Autodesk Inventor part; units mm, degrees
ref_plane "YZ Plane" through (0, 0, 0) normal (1, 0, 0) x (0, 1, 0)
ref_plane "XZ Plane" through (0, 0, 0) normal (0, 1, 0) x (-1, 0, 0)
ref_plane "XY Plane" through (0, 0, 0) normal (0, 0, 1) x (1, 0, 0)
sketch "スケッチ1" plane through (0, 0, 0) normal (0, 0, 1) x (1, 0, 0)
  line L0 (-59, 0) -> (-38, 0)
  line L1 (-38, 0) -> (-38, -21)
  line L2 (-38, -21) -> (-59, -21)
  line L3 (-59, -21) -> (-59, 0)
  line L4 (-61, 2) -> (-36, 2)
  line L5 (-36, 2) -> (-36, -23)
  line L6 (-36, -23) -> (-61, -23)
  line L7 (-61, -23) -> (-61, 2)
  line L8 (-61, -23) -> (0, -23)
  line L9 (0, -23) -> (0, -17)
  line L10 (0, -17) -> (-61, -17)
  line L11 (-61, -17) -> (-61, -23)
  line L12 (-48.5, -23) -> (-85.5, -23)
  line L13 (-85.5, -23) -> (-85.5, -17)
  line L14 (-85.5, -17) -> (-48.5, -17)
  line L15 (-48.5, -17) -> (-48.5, -23)
  line L16 (-85.5, 1) -> (-82.5, 1)
  line L17 (-82.5, 1) -> (-82.5, -23)
  line L18 (-82.5, -23) -> (-85.5, -23)
  line L19 (-85.5, -23) -> (-85.5, 1)
  line L20 (-85.5, -17) -> (-90.7, -17)
  line L21 (-90.7, -17) -> (-90.7, -23)
  line L22 (-90.7, -23) -> (-85.5, -23)
  line L23 (-85.5, -23) -> (-85.5, -17)
  line L24 (-90.7, -23) -> (-93.7, -23)
  line L25 (-93.7, -23) -> (-93.7, 1)
  line L26 (-93.7, 1) -> (-90.7, 1)
  line L27 (-90.7, 1) -> (-90.7, -23)
  point P0 (0, 0)
  point P1 (-61, -10.5)
  point P2 (-59, -10.5)
  point P3 (-48.5, 2)
  point P4 (-48.5, 0)
  point P5 (-36, -17)
  point P6 (-82.5, -17)
  dimension "d0" = 21
  dimension "d1" = 21
  dimension "d4" = 38
  dimension "d5" = 25
  dimension "d6" = 6
  dimension "d31" = 37
  dimension "d33" = 5.2
  dimension "d34" = 3
  dimension "d35" = 18
extrude "押し出し1" add sketch "スケッチ1" along normal blind 8 contours L10 L9 L8 L5
mirror "ミラー2" about plane through (0, -23, 0) normal (1, 0, 0)
sketch "スケッチ17" plane through (0, 0, 0) normal (0, 0, -1) x (-1, 0, 0)
  line L0 (-15, 13) -> (15, 13)
  line L1 (15, 13) -> (15, -17)
  line L2 (15, -17) -> (-15, -17)
  line L3 (-15, -17) -> (-15, 13)
  line L4 (-36, -17) -> (36, -17)
  point P0 (0, 13)
  point P1 (0, 13)
  point P2 (0, -17)
  dimension "d74" = 30
  dimension "d105" = 30
extrude "押し出し16" add sketch "スケッチ17" against normal blind 18
sketch "スケッチ18" plane through (-15, 13, 0) normal (0, 1, 0) x (1, 0, 0)
  line L0 (5, -15.5) -> (25, -15.5)
  line L1 (25, -15.5) -> (25, -2.5)
  line L2 (25, -2.5) -> (5, -2.5)
  line L3 (5, -2.5) -> (5, -15.5)
  line L4 (0, 0) -> (30, 0)
  line L5 (0, 0) -> (0, -18)
  point P0 (15, 0)
  point P1 (15, -2.5)
  point P2 (15, 0)
  point P3 (5, -9)
  point P4 (0, -9)
  dimension "d77" = 20
  dimension "d78" = 13
extrude "押し出し17" cut sketch "スケッチ18" against normal up to surface (30 mm away)
sketch "スケッチ19" plane through (0, 0, 18) normal (0, 0, 1) x (1, 0, 0)
  line L0 (-15, -17) -> (-15, -23)
  line L1 (15, 13) -> (15, -17)
  line L2 (-15, -17) -> (15, -17)
  line L3 (15, -17) -> (15, 11.5)
  line L4 (15, 11.5) -> (-15, 11.5)
  line L5 (-15, 11.5) -> (-15, -17)
  line L6 (15, 13) -> (-15, 13)
  point P0 (0, 0)
  point P1 (-15, 13)
  point P2 (15, -17)
  dimension "d81" = 1.5
extrude "押し出し18" cut sketch "スケッチ19" against normal up to surface (10 mm away)
sketch "スケッチ20" plane through (-15, 11.5, 8) normal (0, 0, 1) x (1, 0, 0)
  line L0 (0, 0) -> (30, 0)
  line L1 (30, -28.5) -> (51, -28.5)
  line L2 (2.5, 0) -> (47.5, 0)
  line L3 (40.5, -28.5) -> (2.5, -28.5)
  line L4 (2.5, -28.5) -> (2.5, 0)
  line L5 (5, 0) -> (5, -28.5)
  line L6 (25, 0) -> (27.5, 0)
  line L7 (27.5, 0) -> (27.5, -28.5)
  line L8 (27.5, -28.5) -> (25, -28.5)
  line L9 (25, -28.5) -> (25, 0)
  line L10 (25, -28.5) -> (25, 0)
  point P0 (15, -11.5)
  point P1 (40.5, -28.5)
  point P2 (25, -15)
  point P3 (5, -15)
  point P4 (51, -28.5)
  point P5 (5, -16)
  point P6 (25, -28.5)
  point P7 (27.5, 0)
  dimension "d85" = 2.5
  dimension "d113" = 2.5
extrude "押し出し19" cut sketch "スケッチ20" against normal up to surface (5.5 mm away) contours L0 L5 L3 L4 | L0 L7 L3 L9
sketch "スケッチ21" plane through (-10, 13, 2.5) normal (0, 0, 1) x (1, 0, 0)
  line L0 (20, 0) -> (20, -1.5)
  line L1 (0, 0) -> (20, 0)
  line L2 (0, 0) -> (0, -1.5)
  line L3 (-2.5, -30) -> (22.5, -30)
  circle A0 centre (10, -15.75) radius 7.5
  line L4 (-5, -1.5) -> (25, -1.5)
  line L5 (-2.5, -30) -> (-2.5, -1.5)
  line L6 (22.5, -30) -> (22.5, -1.5)
  line L7 (22.5, -1.5) -> (20, -1.5)
  line L8 (0, -1.5) -> (-2.5, -1.5)
  line L9 (-2.5, -1.5) -> (-2.5, -30)
  point P0 (0, -2)
  point P1 (10, -1.5)
  point P2 (25, -1.5)
  point P3 (-2.5, -15.75)
  dimension "d89" = 15
extrude "押し出し20" cut sketch "スケッチ21" against normal through all contours A0
sketch "スケッチ26" plane through (-36, -23, 0) normal (0, -1, 0) x (1, 0, 0)
  line L0 (0, 0) -> (72, 0)
  line L1 (72, 0) -> (72, 8)
  line L2 (0, 8) -> (72, 8)
  line L3 (0, 0) -> (0, 8)
  point P0 (36, 0)
extrude "押し出し25" cut sketch "スケッチ26" against normal up to surface (6 mm away)
sketch "スケッチ27" plane through (-15, -17, 0) normal (0, -1, 0) x (1, 0, 0)
  line L0 (-8.5, 8) -> (38.5, 8)
  line L1 (38.5, 8) -> (38.5, 0)
  line L2 (38.5, 0) -> (-8.5, 0)
  line L3 (-8.5, 0) -> (-8.5, 8)
  line L4 (-5, 8) -> (35, 8)
  line L5 (35, 8) -> (35, 0) construction
  line L6 (35, 0) -> (-5, 0)
  line L7 (-5, 0) -> (-5, 8) construction
  line L8 (0, 8) -> (30, 8)
  line L9 (30, 0) -> (0, 0)
  circle A0 centre (-5, 4) radius 1.6
  circle A1 centre (35, 4) radius 1.6
  point P0 (15, 0)
  point P1 (10.6, 8)
  point P2 (15, 0)
  point P3 (15, 0)
  dimension "d108" = 40
  dimension "d109" = 47
  dimension "d110" = 3.2
extrude "押し出し26" add sketch "スケッチ27" against normal blind 3
fillet "フィレット6" radius 6.5 2 edges at (-15, -14, 4) (15, -14, 4)
sketch "スケッチ28" plane through (-15, -14, 0) normal (0, 1, 0) x (1, 0, 0)
  circle A0 centre (-5, -4) radius 1.6
  circle A1 centre (35, -4) radius 1.6
  line L0 (-8.5, -8) -> (38.5, -8)
  line L1 (-8.5, -8) -> (-8.5, 0)
  line L2 (38.5, 0) -> (-8.5, 0)
  line L3 (38.5, 0) -> (38.5, -8)
  circle A2 centre (35, -4) radius 3
  circle A3 centre (-5, -4) radius 3
  point P0 (15, 0)
  dimension "d116" = 6
extrude "押し出し27" cut sketch "スケッチ28" along normal through all contours A0 | A1 | A2 | A3
fillet "フィレット7" radius 4 4 edges at (-23.5, -15.5, 8) (-23.5, -15.5, 0) (23.5, -15.5, 8) (23.5, -15.5, 0)
fillet "フィレット8" radius 9 2 edges at (12.5, -14, 5.25) (-12.5, -14, 5.25)
equation "\"d0\" = d1"
equation "\"d113\" = d85"
properties part number "スイッチセッター"
Geometry: final body of the model. Coordinates: model frame, mm. A direction names the side the tool comes from. Round coordinates to 2 decimals unless told otherwise and drop trailing zeros. Write each loop counter-clockwise with the first axis right and the second up, starting at its lowest first coordinate (ties: lowest second). Pieces come first, ordered by that corner, then holes. Notation, with made-up numbers: M 16.5,47.5 L 51.5,47.5 A17 cw 51.5,74.5 Z; hole C 79,-38 d1. An arc over 180 degrees is marked long. Answer in a Markdown table with one row per item. Add a question column.
(1) Draft query along Y for faces 1 (the face through (22, -14, 4)), 2 (the face through (0, 12, 15.5)), 3 (the face through (-9.794, -11.434, 5.212)). Return one class per face: pulls with the +Y half, pulls with the -Y half, needs draft (parallel to the pull), parting line crosses it, or undercut.
(2) Reachability of faces 4 (the face through (-21.27, -15.52, 3.03)), 5 (the face through (0, 6, 2.5)), 6 (the face through (-12.5, 3, 5)), 7 (the face through (-10, 12, 9)), 8 (the face through (-15, 3, 5)) from +Z, -Z, +X, -X, +Y, -Y: full face, straight path, thin tool, end or side. Return the list, or none.
(3) Ray query, L1, parallel to X at y = 7.5, z = 7; L2, parallel to Z at x = -1, y = 5; L3, parallel to Y at x = 0, z = 1.5. Return the intervals inside material, ascending.
(4) Cut plane B-B, the plane y = -2.75. Return the cut outline in (x, z).
(5) Cut plane C-C, the plane z = 4. Give the number of separate pieces and of enclosed holes in the cut face, then the cut area to 3 significant figures.
(6) Contact query for flat-ended pins moving along their axis: pin 1 (1.5 mm diameter, centred on x = -6, y = 5, fed in from +Z); pin 2 (3 mm diameter, centred on y = -11, z = 7.5, fed in from +X); pin 3 (3 mm diameter, centred on x = 17.5, y = 9, fed in from +Z); pin 4 (4 mm diameter, centred on x = 4, z = 14.5, fed in from -Y). Output: stop coordinate, or through.
(7) Cut plane A-A, the plane x = 0. Return the cut outline in (y, z), then the cut area to 4 significant figures.
(8) Cut plane D-D, the plane z = 8.5. Return the cut outline in (x, y).
Established:
| question | item | result |
|---|---|---|
| 1 | face 1 | pulls with the +Y half |
| 1 | face 2 | needs draft |
| 1 | face 3 | undercut |
| 2 | face 4 | +Y, -Y |
| 2 | face 5 | none |
| 2 | face 6 | +Z |
| 2 | face 7 | +Y |
| 2 | face 8 | +Z, -Z, -X, +Y |
| 3 | L1 | -15 to -12.5, 12.5 to 15 |
| 3 | L2 | 0 to 2.5 |
| 3 | L3 | -17 to -10.25, 4.75 to 13 |
| 4 | outline | M -15,0 L -7.5,0 L -7.5,2.5 L -12.5,2.5 L -12.5,8 L -15,8 Z; M 7.5,0 L 15,0 L 15,8 L 12.5,8 L 12.5,2.5 L 7.5,2.5 Z |
| 5 | separate pieces | 3 |
| 5 | enclosed holes | 0 |
| 5 | area | 312 mm² |
| 6 | pin 1 | z = 2.5 |
| 6 | pin 2 | x = 17.35 |
| 6 | pin 3 | through |
| 6 | pin 4 | y = 11.5 |
| 7 | outline | M -17,0 L -10.25,0 L -10.25,2.5 L -14,2.5 L -14,8 L -17,8 Z; M 4.75,0 L 13,0 L 13,2.5 L 4.75,2.5 Z; M 11.5,15.5 L 13,15.5 L 13,18 L 11.5,18 Z |
| 7 | area | 57.75 mm² |
| 8 | outline | M -15,11.5 L -10,11.5 L -10,13 L -15,13 Z; M 10,11.5 L 15,11.5 L 15,13 L 10,13 Z |
